from build123d import *

# Parameters (mm, degrees)
F3_DEPTH = 1.3
F4_SIZE  = 0.2


with BuildPart() as f1:
    # F0 (on Front) → F1 (revolve)
    with BuildSketch(Plane.XZ):
        Polygon((2.75, 0), (0, 0), (0, -15), (1.5, -15), (1.5, -3), (2.75, -3), align=None)
    revolve(axis=Axis((0, 0, -7.5), (0, 0, -1)))

    # F2 (on face) → F3 (cut)
    with BuildSketch(Plane.XY):
        Polygon((-1.454923, 0), (-0.727461, -1.26), (0.727461, -1.26), (1.454923, 0), (0.727461, 1.26), (-0.727461, 1.26), align=None)
    extrude(amount=-F3_DEPTH, mode=Mode.SUBTRACT)

    # F4
    f4_edges = [f1.edges().sort_by_distance(p)[0] for p in [
        (-2.75, 0, -3),
        (-2.75, 0, 0),
        (2.75, 0, -1.5),
        (-1.5, 0, -15),
    ]]
    chamfer(f4_edges, length=F4_SIZE)


solid = f1.part
Design review of the part built by this model. Coordinates are the model's own, in mm. A direction names the side the tool comes from. Round coordinates to 2 decimals unless told otherwise and drop trailing zeros. Write each loop counter-clockwise with the first axis right and the second up, starting at its lowest first coordinate (ties: lowest second). Pieces come first, ordered by that corner, then holes.
Item 1: Consider section C-C on z = -6.5. Give the boundary of the cut face in (x, y).
Item 2: Consider section B-B on z = -1.5. Give the boundary of the cut face in (x, y), and give its area (3 significant figures).
Item 3: Draft analysis for pull direction X (two halves, no side actions). For faces 4 (the flat face through (-1.096, -0.621, -0.641)), 5 (the cylindrical face through (-1.5, -0.07, -8.82)), 6 (the flat face through (1.1, 1.1, 0)), state which applies: released by +X, released by -X, zero draft, split by the parting line, or undercut.
Item 4: For pin 1 Ø3 at (x, y) = (-0.5, -0.5) entering from +Z; pin 2 Ø3 at (x, z) = (-0.5, -12.5) entering from +Y; pin 3 Ø1 at (y, z) = (-0.5, -13.5) entering from -X, all flat-tipped, find the tip position at first contact; note any pin that passes through.
Item 5: Wall thickness on L1, parallel to Z at x = 1.95, y = 0.75; L2, parallel to X at y = -0.35, z = -4; L3, parallel to X at y = 0.75, z = -10.75: over which ranges is each line inside the solid? List them lowest first.
Item 6: Consider section A-A on x = 0. Give the boundary of the cut face in (y, z).
Item 7: For faces 1 (the flat face through (0, -1.26, -1)), 2 (the flat face through (0, 0, -15)), 3 (the flat face through (-2, 0, -3)), list the 3-axis set-ups (+Z, -Z, +X, -X, +Y, -Y) from which the entire face can be reached by the end or side of a thin tool; tool diameter is ignored.
Check values:
1. outline: circle Ø3 at (0, 0)
2. outline: circle Ø5.5 at (0, 0)
2. area: 23.8 mm2
3. face 4: undercut
3. face 5: split by the parting line
3. face 6: zero draft
4. pin 1: stops at z = 0
4. pin 2: stops at y = 1.5
4. pin 3: stops at x = -1.5
5. L1: z = -3 to 0
5. L2: x = -1.46 to 1.46
5. L3: x = -1.3 to 1.3
6. outline: (-2.75, -2.8) - (-2.55, -3) - (-1.5, -3) - (-1.5, -14.8) - (-1.3, -15) - (1.3, -15) - (1.5, -14.8) - (1.5, -3) - (2.55, -3) - (2.75, -2.8) - (2.75, -0.2) - (2.55, 0) - (1.26, 0) - (1.26, -1.3) - (-1.26, -1.3) - (-1.26, 0) - (-2.55, 0) - (-2.75, -0.2) - close
7. face 1: +Z
7. face 2: -Z, +X, -X, +Y, -Y
7. face 3: -Z
